Geometry check sheet. Reference: the model listing, model coordinates, mm. A direction names the side the tool comes from. Give positions to 0.01 mm unless a question says otherwise; leave off trailing zeros. Loops run counter-clockwise (first coordinate to the right, second up) from the corner with the lowest first, then second, coordinate; pieces in that order, holes last. Notation, with made-up numbers: (11, 40) - (45, 40) arc R26 cw to (45, 77) - close; hole circle Ø2 at (-30, 20). An arc over 180 degrees is marked (long way). Use a Markdown table: item, result. Add a question column.
1. Depth check by flat-ended pin: P1, Ø1.5, axis at x = 41, z = 2, coming from the -Y side; P2, Ø0.9, axis at x = 46.5, z = 3.5, coming from the +Y side; P3, Ø2, axis at x = 43.5, y = -42.5, coming from the -Z side. Enter the tip coordinate at first touch or a pass-through.
2. Set-up check for faces 1 (the flat face through (45, -36, 3)), 2 (the flat face through (45, -44, 3)): record each of +Z, -Z, +X, -X, +Y, -Y from which the full face is reachable in a straight line by a thin tool's end or side.
3. Cross-section at A-A on z = 3.4. Enter the section's corners in (x, y), and give its area (3 significant figures).
4. Material ranges on L1, parallel to Y at x = 43.25, z = 3 (3 decimals); L2, parallel to Y at x = 42, z = 3.35; L3, parallel to Y at x = 40.75, z = 4.45, recorded low to high.
5. Cross-section at C-C on y = -41. Enter the section's corners in (x, z) (3 decimals).
6. Draft check along Y on faces 3 (the cylindrical face through (43.975, -39.706, 3.17)), 4 (the flat face through (40.337, -40.291, 1.625)), 5 (the flat face through (42, -33.5, 3)), 6 (the flat face through (43, -39, 0)). Enter one of: pulls with the +Y half, pulls with the -Y half, needs draft (parallel to the pull), parting line crosses it, or undercut.
7. Cross-section at B-B on x = 42. Enter the section's corners in (y, z) (3 decimals).
8. Cross-section at D-D on x = 45.25. Enter the section's corners in (y, z) (3 decimals).
from build123d import *

# Parameters (mm, degrees)
SKETCH1_R           = 1.55
BOSS_EXTRUDE1_DEPTH = 6
SKETCH3_R           = 1.305
CUT_EXTRUDE3_DEPTH  = 10


with BuildPart() as part:
    # Sketch1 → Boss-Extrude1 (new body)
    with BuildSketch(Plane.XY):
        Polygon((48, -38), (45, -38), (45, -33.5), (39, -33.5), (39, -38), (42.5, -44), (48, -44), align=None)
        with Locations((42, -36.5)):
            Circle(SKETCH1_R, mode=Mode.SUBTRACT)
    extrude(amount=BOSS_EXTRUDE1_DEPTH)

    # Sketch3 → Cut-Extrude3 (cut, through all)
    with BuildSketch(Plane(origin=(48, 0, 0), x_dir=(0, 0, -1), z_dir=(1, 0, 0))):
        with Locations((-3, -41)):
            Circle(SKETCH3_R)
    extrude(amount=-CUT_EXTRUDE3_DEPTH, mode=Mode.SUBTRACT)


solid = part.part
Values found:
| question | item | result |
|---|---|---|
| 1 | P1 | stops at y = -42.71 |
| 1 | P2 | stops at y = -38 |
| 1 | P3 | stops at z = 0 |
| 2 | face 1 | +Z, -Z, +X, +Y |
| 2 | face 2 | +Z, -Z, +X, -X, -Y |
| 3 | outline | (39, -38) - (40.03, -39.76) - (48, -39.76) - (48, -38) - (45, -38) - (45, -33.5) - (39, -33.5) - close; (41.47, -42.24) - (42.5, -44) - (48, -44) - (48, -42.24) - close; hole circle Ø3.1 at (42, -36.5) |
| 3 | area | 44.9 mm2 |
| 4 | L1 | y = -44 to -42.305, -39.695 to -37.417, -35.583 to -33.5 |
| 4 | L2 | y = -43.14 to -42.26, -39.74 to -38.05, -34.95 to -33.5 |
| 4 | L3 | y = -41 to -37.42, -35.58 to -33.5 |
| 5 | outline | (40.75, 0) - (48, 0) - (48, 1.695) - (40.75, 1.695) - close; (40.75, 4.305) - (48, 4.305) - (48, 6) - (40.75, 6) - close |
| 6 | face 3 | undercut |
| 6 | face 4 | pulls with the -Y half |
| 6 | face 5 | pulls with the +Y half |
| 6 | face 6 | needs draft |
| 7 | outline | (-43.143, 0) - (-38.05, 0) - (-38.05, 6) - (-43.143, 6) - close; (-34.95, 0) - (-33.5, 0) - (-33.5, 6) - (-34.95, 6) - close; hole circle Ø2.61 at (-41, 3) |
| 8 | outline | (-44, 0) - (-38, 0) - (-38, 6) - (-44, 6) - close; hole circle Ø2.61 at (-41, 3) |
